Input: dimensioned drawing with shaded views. Units: mm. Origin: part minimum x, y, z. Give positions to 0.01 mm unless a question says otherwise; leave off trailing zeros. Write each loop counter-clockwise with the first axis right and the second up, starting at its lowest first coordinate (ties: lowest second). Pieces come first, ordered by that corner, then holes. Notation, with made-up numbers: (8.5, 63.5) -> (46.5, 63.5) arc R15 cw to (46.5, 70.5) -> close; hole circle Ø3 at (-40, 54.25). An arc over 180 degrees is marked (long way). Answer as a JSON object with one key per item and string values.
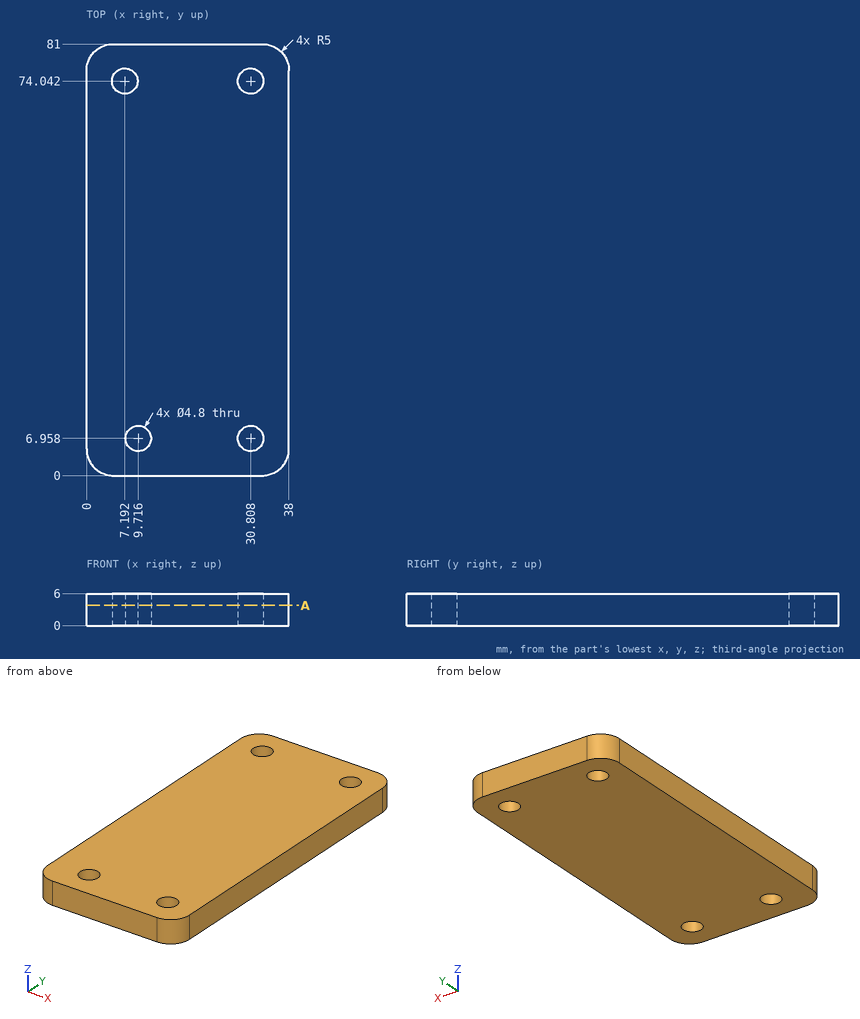
Q1. First-contact query: P1, Ø4.5, axis at x = 30.81, y = 74.04, coming from the +Z side. Flat tip, straight axial feed; report the tip coordinate or a pass-through.
Values:
{"P1": "through"}
Q2. Material intervals for L1, parallel to Y at x = 30, z = 0.6; L2, parallel to Y at x = 29.5, z = 5.7 (1 decimal); L3, parallel to Y at x = 5, z = 1.85 (1 decimal), sorted ascending. Write a range as from..to.
Values:
{"L1": "0..4.7, 9.22..71.78, 76.3..81", "L2": "0..4.9, 9..72, 76.1..81", "L3": "0..73.1, 75..81"}
Q3. Cut plane A-A (z = 3.8). Return the cut outline in (x, y), and give its area (3 significant figures).
Values:
{"outline": "(0, 5) arc R5 ccw to (5, 0) -> (33, 0) arc R5 ccw to (38, 5) -> (38, 76) arc R5 ccw to (33, 81) -> (5, 81) arc R5 ccw to (0, 76) -> close; hole circle Ø4.8 at (7.19, 74.04); hole circle Ø4.8 at (9.72, 6.96); hole circle Ø4.8 at (30.81, 6.96); hole circle Ø4.8 at (30.81, 74.04)", "area": "2,980 mm²"}
